Job drawing, mm, ordinate dimensions from the low corner. One solid piece. Coordinates: 2 decimals unless noted, no trailing zeros. Write each loop counter-clockwise with the first axis right and the second up, starting at its lowest first coordinate (ties: lowest second). Pieces come first, ordered by that corner, then holes. Notation, with made-up numbers: (25.25, -4) -> (48.25, -4) arc R28 cw to (48.25, 33) -> close; hole circle Ø6 at (81.5, -21.5). An arc over 180 degrees is marked (long way). One line per question, with ' | ' between items. Start each with the question number.
Item 1: Pin check, flat tips, straight feed: pin 1 (2 mm diameter, centred on x = 9.5, z = 2, fed in from -Y); pin 2 (3.5 mm diameter, centred on x = 12.5, y = 63, fed in from -Z). Stop position of each tip, or through.
Item 2: Saw through at B-B (z = 2.35). List the corners of the cut face in (x, y).
Item 3: Saw through at C-C (y = 63). List the corners of the cut face in (x, z).
Item 4: Probe probe 1 along Y at (x, z) = (12.5, 2.75); probe 2 along X at (y, z) = (73, 1.15); probe 3 along Y at (x, z) = (8, 4.65). List the from-to ranges inside material, lowest first. Write a range as [from, to].
Item 5: Saw through at D-D (x = 7.5). List the corners of the cut face in (y, z), and give its area (3 significant figures).
Item 6: Saw through at A-A (x = 12.5). List the corners of the cut face in (y, z).
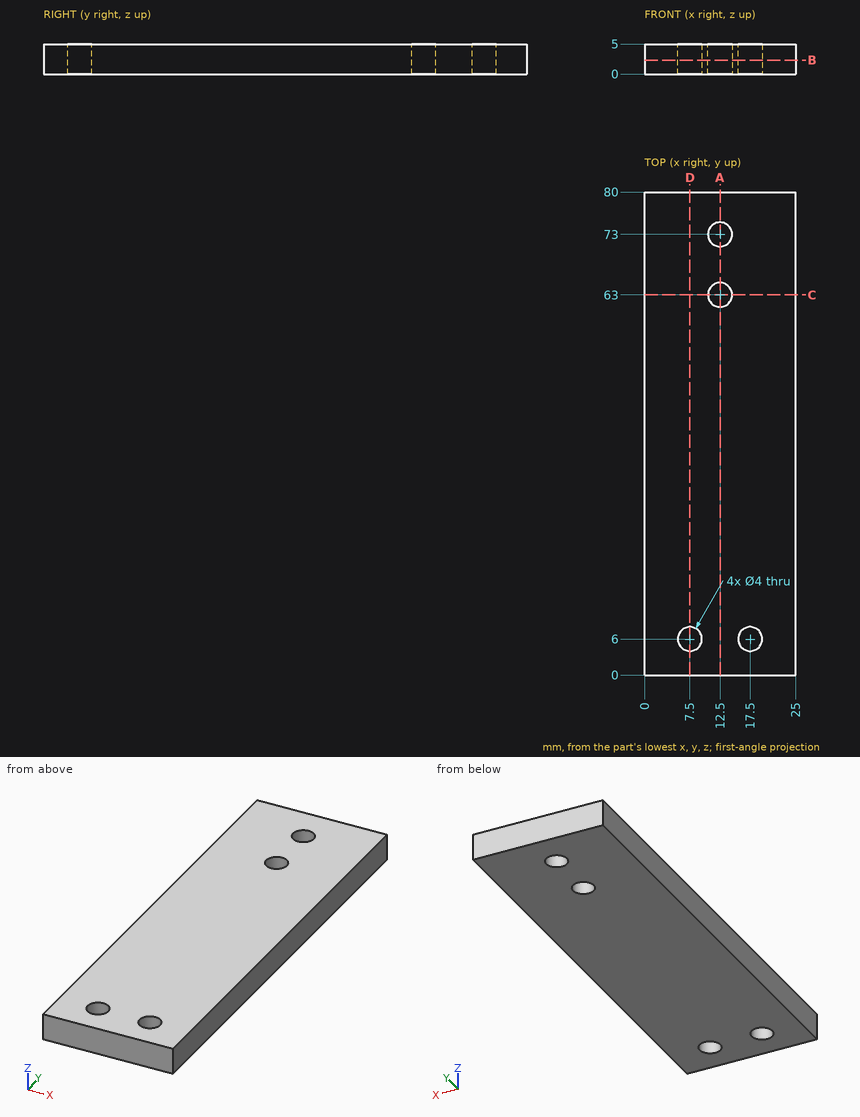
From the geometry:
1) pin 1: y = 0 | pin 2: through
2) outline: (0, 0) -> (25, 0) -> (25, 80) -> (0, 80) -> close; hole circle Ø4 at (7.5, 6); hole circle Ø4 at (12.5, 63); hole circle Ø4 at (12.5, 73); hole circle Ø4 at (17.5, 6)
3) outline: (0, 0) -> (10.5, 0) -> (10.5, 5) -> (0, 5) -> close; (14.5, 0) -> (25, 0) -> (25, 5) -> (14.5, 5) -> close
4) probe 1: [0, 61], [65, 71], [75, 80] | probe 2: [0, 10.5], [14.5, 25] | probe 3: [0, 4.06], [7.94, 80]
5) outline: (0, 0) -> (4, 0) -> (4, 5) -> (0, 5) -> close; (8, 0) -> (80, 0) -> (80, 5) -> (8, 5) -> close | area: 380 mm2
6) outline: (0, 0) -> (61, 0) -> (61, 5) -> (0, 5) -> close; (65, 0) -> (71, 0) -> (71, 5) -> (65, 5) -> close; (75, 0) -> (80, 0) -> (80, 5) -> (75, 5) -> close
